Can you work these out from the model? Positions are in its coordinate system, mm. Face numbers are marked on the shaded views. A direction names the side the tool comes from. Round coordinates to 2 decimals unless told otherwise and drop trailing zeros. Loops run counter-clockwise (first coordinate to the right, second up) from the corner with the lowest first, then second, coordinate; pieces in that order, holes last. Notation, with made-up numbers: M 33.25,-4 L 55.25,-4 A30 ccw 55.25,33 Z; hole C -26,0 d8. An arc over 180 degrees is marked long. Return JSON: item names as keys, results as strings.
```python
from build123d import *
from build123d.topology import SkipClean

# Parameters (mm, degrees)
SKETCH1_R           = 21.2
SKETCH1_R_2         = 17.5
BOSS_EXTRUDE1_DEPTH = 5
BOSS_EXTRUDE2_START = -5
SKETCH2_R           = 21.2
BOSS_EXTRUDE2_DEPTH = 5
BOSS_EXTRUDE3_START = 25
BOSS_EXTRUDE3_DEPTH = 25
SKETCH5_R           = 5
CUT_EXTRUDE1_DEPTH  = 98.012576504
SKETCH7_R           = 8.1
CUT_EXTRUDE2_DEPTH  = 3
SKETCH10_R          = 1.65
CUT_EXTRUDE3_DEPTH  = 23
SKETCH11_R          = 1.6
CUT_EXTRUDE4_DEPTH  = 33
SKETCH12_W          = 20.5
SKETCH12_H          = 5
CUT_EXTRUDE5_DEPTH  = 99.419713472
SKETCH13_R          = 1.6
CUT_EXTRUDE6_DEPTH  = 98.012576504
SKETCH14_R          = 2.8
CUT_EXTRUDE7_DEPTH  = 3
BOSS_EXTRUDE4_START = 5
BOSS_EXTRUDE4_DEPTH = 5
CUT_EXTRUDE9_DEPTH  = 108.101633974
SKETCH23_R          = 1
CUT_EXTRUDE11_DEPTH = 1


with BuildPart() as part:
    # Sketch1 → Boss-Extrude1 (new body)
    with BuildSketch(Plane.XY):
        Circle(SKETCH1_R)
        Circle(SKETCH1_R_2, mode=Mode.SUBTRACT)
    extrude(amount=BOSS_EXTRUDE1_DEPTH)

    # Sketch2 → Boss-Extrude2 (add)
    with BuildSketch(Plane.XY.offset(5).offset(BOSS_EXTRUDE2_START)):
        with BuildLine():
            Line((26.2, 0), (26.2, -90))
            Line((26.2, -90), (-26.2, -90))
            Line((-26.2, -90), (-26.2, 0))
            ThreePointArc((-26.2, 0), (0, 26.2), (26.2, 0))
        make_face()
        Circle(SKETCH2_R, mode=Mode.SUBTRACT)
    extrude(amount=BOSS_EXTRUDE2_DEPTH)

    # Sketch4 → Boss-Extrude3 (add)
    with BuildSketch(Plane(origin=(0, 0, 0), x_dir=(-1, 0, 0), z_dir=(0, 0, -1)).offset(BOSS_EXTRUDE3_START)):
        with BuildLine():
            Line((-26.2, 0), (-26.2, -90))
            Line((-26.2, -90), (26.2, -90))
            Line((26.2, -90), (26.2, 0))
            ThreePointArc((26.2, 0), (0, 26.2), (-26.2, 0))
        make_face()
        with BuildLine():
            Line((-21.2, 0), (-21.2, -85))
            Line((-21.2, -85), (21.2, -85))
            Line((21.2, -85), (21.2, 0))
            ThreePointArc((21.2, 0), (0, 21.2), (-21.2, 0))
        make_face(mode=Mode.SUBTRACT)
    extrude(amount=-BOSS_EXTRUDE3_DEPTH)

    # Sketch5 → Cut-Extrude1 (cut, through all)
    with BuildSketch(Plane(origin=(0, 0, 0), x_dir=(-1, 0, 0), z_dir=(0, 0, -1))):
        with Locations((12.995105527, -36.242762456)):
            Circle(SKETCH5_R)
    extrude(amount=-CUT_EXTRUDE1_DEPTH, mode=Mode.SUBTRACT)

    # Sketch7 → Cut-Extrude2 (cut)
    with BuildSketch(Plane(origin=(0, 0, 0), x_dir=(-1, 0, 0), z_dir=(0, 0, -1))):
        with Locations((12.995105527, -36.242762456)):
            Circle(SKETCH7_R)
    extrude(amount=-CUT_EXTRUDE2_DEPTH, mode=Mode.SUBTRACT)

    # Sketch10 → Cut-Extrude3 (cut)
    with BuildSketch(Plane.XZ.offset(90)):
        with Locations(Location((15.5, -5.5, 0), (0, 0, 270))):
            Circle(SKETCH10_R)
        with Locations((15.5, -36.5)):
            Circle(SKETCH10_R)
        with Locations((-15.5, -36.5)):
            Circle(SKETCH10_R)
        with Locations(Location((-15.5, -5.5, 0), (0, 0, 270))):
            Circle(SKETCH10_R)
    extrude(amount=-CUT_EXTRUDE3_DEPTH, mode=Mode.SUBTRACT)

    # Sketch11 → Cut-Extrude4 (cut)
    with BuildSketch(Plane(origin=(0, 0, -25), x_dir=(-1, 0, 0), z_dir=(0, 0, -1))):
        with Locations((-23.7, -87.5)):
            Circle(SKETCH11_R)
        with Locations((23.7, -87.5)):
            Circle(SKETCH11_R)
        with Locations((0, 23.7)):
            Circle(SKETCH11_R)
        with Locations((23.7, 0)):
            Circle(SKETCH11_R)
        with Locations((-23.7, 0)):
            Circle(SKETCH11_R)
    extrude(amount=-CUT_EXTRUDE4_DEPTH, mode=Mode.SUBTRACT)

    # Sketch12 → Cut-Extrude5 (cut, through all)
    with BuildSketch(Plane(origin=(0, 0, -25), x_dir=(-1, 0, 0), z_dir=(0, 0, -1))):
        with Locations((0, -90)):
            Rectangle(SKETCH12_W, SKETCH12_H)
    extrude(amount=-CUT_EXTRUDE5_DEPTH, mode=Mode.SUBTRACT)

    # Sketch13 → Cut-Extrude6 (cut, through all)
    with BuildSketch(Plane(origin=(0, 0, 0), x_dir=(-1, 0, 0), z_dir=(0, 0, -1))):
        with Locations((-2.493558329, -26.106401349)):
            Circle(SKETCH13_R)
    extrude(amount=-CUT_EXTRUDE6_DEPTH, mode=Mode.SUBTRACT)

    # Sketch14 → Cut-Extrude7 (cut)
    with BuildSketch(Plane.XY.offset(5)):
        with Locations((2.493558329, -26.106401349)):
            Circle(SKETCH14_R)
    extrude(amount=-CUT_EXTRUDE7_DEPTH, mode=Mode.SUBTRACT)

    # Sketch15 → Boss-Extrude4 (add)
    with SkipClean():  # the faces are left unmerged after this step: merging them gives an invalid solid
        with BuildSketch(Plane(origin=(0, 0, 0), x_dir=(-1, 0, 0), z_dir=(0, 0, -1)).offset(BOSS_EXTRUDE4_START)):
            with BuildLine():
                Line((21.2, -11.670475569), (21.2, 0))
                ThreePointArc((21.2, 0), (0, -21.2), (-21.2, 0))
                Line((-21.2, 0), (-21.2, -11.670475569))
                ThreePointArc((-21.2, -11.670475569), (0, -24.2), (21.2, -11.670475569))
            make_face()
        extrude(amount=-BOSS_EXTRUDE4_DEPTH)

    # Sketch19 → Cut-Extrude9 (cut, through all)
    with SkipClean():  # the faces are left unmerged after this step: merging them gives an invalid solid
        with BuildSketch(Plane(origin=(26.2, 0, 0), x_dir=(0, 0, -1), z_dir=(1, 0, 0))):
            with BuildLine():
                Line((0, -61.002267957), (0, -62.755091356))
                ThreePointArc((0, -62.755091356), (0.66664465, -64.002295774), (2.074025149, -64.140910655))
                Line((2.074025149, -64.140910655), (19.074025149, -57.099280094))
                ThreePointArc((19.074025149, -57.099280094), (19.747204418, -56.546816145), (20, -55.713460796))
                Line((20, -55.713460796), (20, -53.960637397))
                ThreePointArc((20, -53.960637397), (19.33335535, -52.713432978), (17.925974851, -52.574818098))
                Line((17.925974851, -52.574818098), (0.925974851, -59.616448658))
                ThreePointArc((0.925974851, -59.616448658), (0.252795582, -60.168912607), (0, -61.002267957))
            make_face()
            with BuildLine():
                Line((0, -71.002267957), (0, -72.755091356))
                ThreePointArc((0, -72.755091356), (0.66664465, -74.002295774), (2.074025149, -74.140910655))
                Line((2.074025149, -74.140910655), (19.074025149, -67.099280094))
                ThreePointArc((19.074025149, -67.099280094), (19.747204418, -66.546816145), (20, -65.713460796))
                Line((20, -65.713460796), (20, -63.960637397))
                ThreePointArc((20, -63.960637397), (19.33335535, -62.713432978), (17.925974851, -62.574818098))
                Line((17.925974851, -62.574818098), (0.925974851, -69.616448658))
                ThreePointArc((0.925974851, -69.616448658), (0.252795582, -70.168912607), (0, -71.002267957))
            make_face()
            with BuildLine():
                Line((0, -51.002267957), (0, -52.755091356))
                ThreePointArc((0, -52.755091356), (0.66664465, -54.002295774), (2.074025149, -54.140910655))
                Line((2.074025149, -54.140910655), (19.074025149, -47.099280094))
                ThreePointArc((19.074025149, -47.099280094), (19.747204418, -46.546816145), (20, -45.713460796))
                Line((20, -45.713460796), (20, -43.960637397))
                ThreePointArc((20, -43.960637397), (19.33335535, -42.713432978), (17.925974851, -42.574818098))
                Line((17.925974851, -42.574818098), (0.925974851, -49.616448658))
                ThreePointArc((0.925974851, -49.616448658), (0.252795582, -50.168912607), (0, -51.002267957))
            make_face()
            with BuildLine():
                Line((0, -41.002267957), (0, -42.755091356))
                ThreePointArc((0, -42.755091356), (0.66664465, -44.002295774), (2.074025149, -44.140910655))
                Line((2.074025149, -44.140910655), (19.074025149, -37.099280094))
                ThreePointArc((19.074025149, -37.099280094), (19.747204418, -36.546816145), (20, -35.713460796))
                Line((20, -35.713460796), (20, -33.960637397))
                ThreePointArc((20, -33.960637397), (19.33335535, -32.713432978), (17.925974851, -32.574818098))
                Line((17.925974851, -32.574818098), (0.925974851, -39.616448658))
                ThreePointArc((0.925974851, -39.616448658), (0.252795582, -40.168912607), (0, -41.002267957))
            make_face()
        extrude(amount=-CUT_EXTRUDE9_DEPTH, mode=Mode.SUBTRACT)

    # Sketch23 → Cut-Extrude11 (cut)
    with SkipClean():  # the faces are left unmerged after this step: merging them gives an invalid solid
        with BuildSketch(Plane.XY.offset(5)):
            with Locations((-15.2, -55.029144675)):
                Circle(SKETCH23_R)
            with Locations((-23.202663328, -60.148459048)):
                Circle(SKETCH23_R)
        extrude(amount=-CUT_EXTRUDE11_DEPTH, mode=Mode.SUBTRACT)


solid = part.part
```
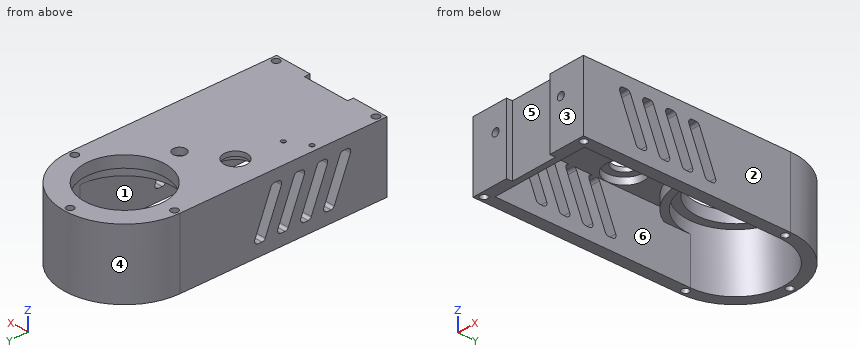
Q1. Suppose I cut it at A-A, the plane x = 3. Please give me the cut outline in (y, z), plus the area to 3 significant figures.
Results:
{"outline": "M -87.5,-25 L -85,-25 L -85,0 L -27.62,0 L -27.62,2 L -28.86,2 L -28.86,5 L -87.5,5 Z; M -24.59,0 L -24.01,0 L -24.01,-5 L -20.99,-5 L -20.99,0 L -17.24,0 L -17.24,5 L -23.35,5 L -23.35,2 L -24.59,2 Z; M 17.24,0 L 20.99,0 L 20.99,-25 L 26.03,-25 L 26.03,5 L 17.24,5 Z", "area": "576 mm2"}
Q2. Suppose I cut it at C-C, the plane y = 23.7. Please give me the cut outline in (x, z), plus the area to 3 significant figures.
Results:
{"outline": "M -11.17,-25 L -1.6,-25 L -1.6,5 L -11.17,5 Z; M 1.6,-25 L 11.17,-25 L 11.17,5 L 1.6,5 Z", "area": "574 mm2"}
Q3. Thinking about a two-plate mould opening in X: for the marked faces 1, 2 and 3, which applies, pulls with the +X half, pulls with the -X half, needs draft (parallel to the pull), parting line crosses it, or undercut?
Results:
{"face 1": "undercut", "face 2": "pulls with the +X half", "face 3": "needs draft"}
Q4. If I drill on line 1 along X through (y, z) = (-72, -19.25); line 2 along Y through (x, z) = (0, 1.15); line 3 along Y through (x, z) = (0, -12.75), over which ranges is the centre line in solid material (lowest first)?
Results:
{"line 1": "x = -26.2 to -21.2, 21.2 to 26.2", "line 2": "y = -87.5 to -17.5, 17.5 to 22.1, 25.3 to 26.2", "line 3": "y = -87.5 to -85, 21.2 to 22.1, 25.3 to 26.2"}
Q5. Suppose I cut it at D-D, the plane z = -8.75. State how many separate pieces and enclosed holes the cut face has, plus the area to 3 significant figures.
Results:
{"separate pieces": "8", "enclosed holes": "5", "area": "1,190 mm2"}
Q6. I'm going to push flat-ended pins straight in: pin 1 Ø7.5 at (x, y) = (7.5, -13) entering from -Z; pin 2 Ø11.5 at (x, y) = (-13, -36.24) entering from -Z; pin 3 Ø1.5 at (y, z) = (5.5, -15) entering from +X. Where does each tip first touch, or does it pass through?
Results:
{"pin 1": "stops at z = 0", "pin 2": "stops at z = 3", "pin 3": "stops at x = 25.77"}
Q7. Suppose I cut it at B-B, the plane y = -79. Please give me the cut outline in (x, z), plus the area to 3 significant figures.
Results:
{"outline": "M -26.2,-25 L -21.2,-25 L -21.2,0 L 21.2,0 L 21.2,-25 L 26.2,-25 L 26.2,5 L -26.2,5 Z", "area": "512 mm2"}
Q8. On a 3-axis mill with a long thin cutter (end or side, diameter ignored), from which of +Z, -Z, +X, -X, +Y, -Y can I reach the whole of each face in a straight line? I mean the marked faces 4, 5 and 6. Say none if no direction works.
Results:
{"face 4": "+Z, -Z, +Y", "face 5": "+Z, -Z, -Y", "face 6": "-Z"}
